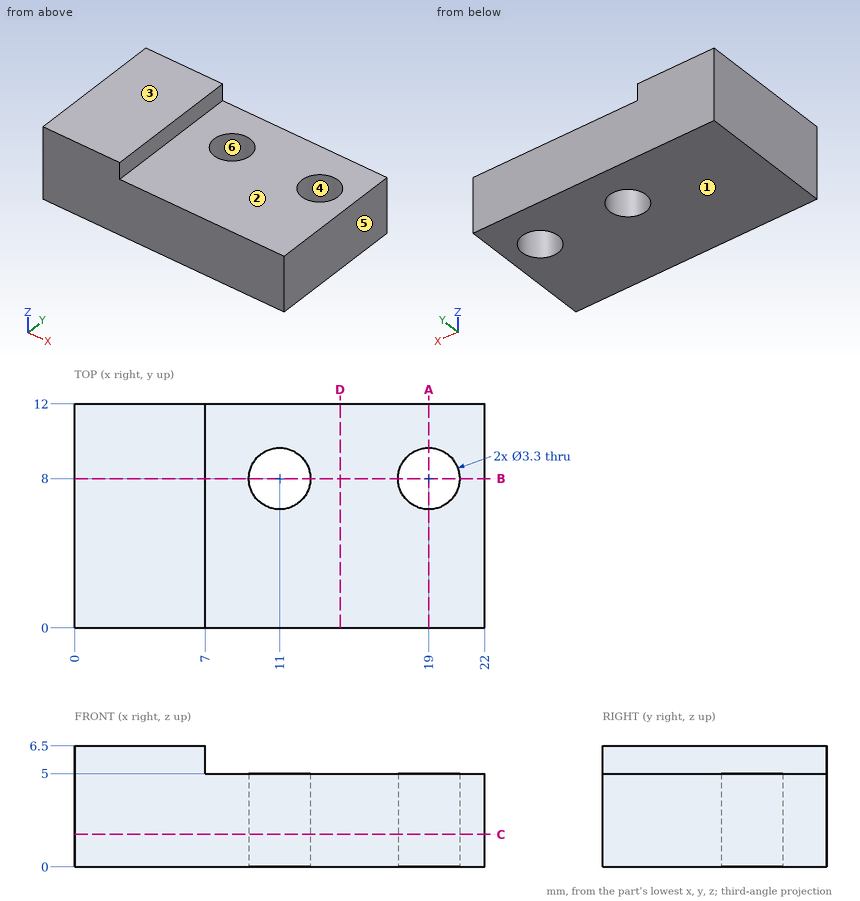
Design review of the part shown in the three views and the two pictorial views. Dimensions are in mm from the part's minimum x, y and z. A direction names the side the tool comes from. Round coordinates to 2 decimals unless told otherwise and drop trailing zeros. Order: outer loops, then holes, each group sorted by start corner. A loop starts at its lowest first (then second) coordinate and runs counter-clockwise, first axis right, second up. Notation, with made-up numbers: (43, -4.75) - (91, -4.75) arc R21 cw to (91, 20.25) - close; hole circle Ø8 at (68.5, 67.5). An arc over 180 degrees is marked (long way). Answer in a Markdown table with one row per item.
(1) Mouldability with a two-part tool opening along X and no side actions: class the marked faces 3, 4, 5 and 6 as released by +X, released by -X, zero draft, split by the parting line, or undercut.
Result set:
| item | result |
|---|---|
| face 3 | zero draft |
| face 4 | undercut |
| face 5 | released by +X |
| face 6 | undercut |
(2) Take a section at B-B on y = 8. Write out the cut boundary in (x, z), plus the area to 3 significant figures.
Result set:
| item | result |
|---|---|
| outline | (0, 0) - (9.35, 0) - (9.35, 5) - (7, 5) - (7, 6.5) - (0, 6.5) - close; (12.65, 0) - (17.35, 0) - (17.35, 5) - (12.65, 5) - close; (20.65, 0) - (22, 0) - (22, 5) - (20.65, 5) - close |
| area | 87.5 mm2 |
(3) Machinability: for the marked faces 1 and 2, which of the approach directions +Z, -Z, +X, -X, +Y, -Y give a long, thin tool a straight path to every point of the face, cutting with its end or side? Answer none if there is none.
Result set:
| item | result |
|---|---|
| face 1 | -Z, +X, -X, +Y, -Y |
| face 2 | +Z, +X, +Y, -Y |
(4) For line 1 (Y direction, x = 19, z = 3.6); line 2 (X direction, y = 7.25, z = 2); line 3 (X direction, y = 9, z = 4.75), list the stretches that pass through material, from the lowest coordinate up. Write a range as from..to.
Result set:
| item | result |
|---|---|
| line 1 | y = 0..6.35, 9.65..12 |
| line 2 | x = 0..9.53, 12.47..17.53, 20.47..22 |
| line 3 | x = 0..9.69, 12.31..17.69, 20.31..22 |
(5) Take a section at A-A on x = 19. Write out the cut boundary in (y, z), plus the area to 3 significant figures.
Result set:
| item | result |
|---|---|
| outline | (0, 0) - (6.35, 0) - (6.35, 5) - (0, 5) - close; (9.65, 0) - (12, 0) - (12, 5) - (9.65, 5) - close |
| area | 43.5 mm2 |
(6) Take a section at D-D on x = 14.25. Write out the cut boundary in (y, z), plus the area to 3 significant figures.
Result set:
| item | result |
|---|---|
| outline | (0, 0) - (12, 0) - (12, 5) - (0, 5) - close |
| area | 60.0 mm2 |
(7) Take a section at C-C on z = 1.75. Write out the cut boundary in (x, y).
Result set:
| item | result |
|---|---|
| outline | (0, 0) - (22, 0) - (22, 12) - (0, 12) - close; hole circle Ø3.3 at (11, 8); hole circle Ø3.3 at (19, 8) |
